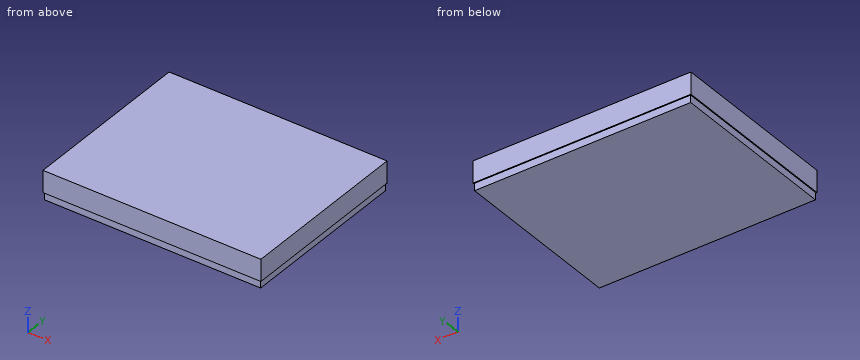
from build123d import *

# Parameters (mm, degrees)
F0_W     = 762
F0_H     = 609.6
F1_DEPTH = 101.6
F2_W     = 755.65
F2_H     = 603.25
F3_DEPTH = 25.4


with BuildPart() as f1:
    # F0 (on Top) → F1 (new body)
    with BuildSketch(Plane.XY):
        with Locations((381, 304.8)):
            Rectangle(F0_W, F0_H)
    extrude(amount=F1_DEPTH)

    # F2 (on face) → F3 (cut)
    with BuildSketch(Plane(origin=(0, 0, 0), x_dir=(1, 0, 0), z_dir=(0, 0, -1))):
        Polygon((762, 0), (0, 0), (0, -3.175), (0, -606.425), (0, -609.6), (762, -609.6), (762, -606.425), (762, -3.175), align=None)
        with Locations((381, -304.8)):
            Rectangle(F2_W, F2_H, mode=Mode.SUBTRACT)
    extrude(amount=-F3_DEPTH, mode=Mode.SUBTRACT)


solid = f1.part
Geometry: final body of the model. Coordinates: model frame, mm. Coordinates: 2 decimals unless noted, no trailing zeros. Loops run counter-clockwise (first coordinate to the right, second up) from the corner with the lowest first, then second, coordinate; pieces in that order, holes last. Notation, with made-up numbers: (-40, 85.25) - (-30, 85.25) arc R24 cw to (-30, 111.25) - close; hole circle Ø7 at (1.5, 57). An arc over 180 degrees is marked (long way). One line per question, with ' | ' between items. Start each with the question number.
(1) Ray query, L1, parallel to X at y = 493.5, z = 8 (3 decimals); L2, parallel to Y at x = 728, z = 10 (3 decimals). Return the intervals inside material, ascending. Write a range as from..to.
(2) First-contact query: pin 1 (8 mm diameter, centred on x = 229.5, y = 365.5, fed in from -Z); pin 2 (7.5 mm diameter, centred on y = 430.5, z = 17.5, fed in from -X) (3 decimals); pin 3 (2 mm diameter, centred on x = 162.5, z = 21, fed in from +Y) (3 decimals); pin 4 (7.5 mm diameter, centred on x = 218.5, z = 19, fed in from -Y) (3 decimals). Flat tips, straight axial feed; report the tip coordinate or a pass-through.
(3) Cut plane A-A on z = 14. Output: boundary loops of the cut face in (x, y) (3 decimals).
Here are the results:
1) L1: 3.175..758.825 | L2: 3.175..606.425
2) pin 1: z = 0 | pin 2: x = 3.175 | pin 3: y = 606.425 | pin 4: y = 3.175
3) outline: (3.175, 3.175) - (758.825, 3.175) - (758.825, 606.425) - (3.175, 606.425) - close
